```python
from build123d import *

# Parameters (mm, degrees)
SZKIC1_W                    = 90
SZKIC1_H                    = 56
DODANIE_WYCI_GNI_CIE1_DEPTH = 3
SZKIC2_W                    = 90
SZKIC2_H                    = 3
DODANIE_WYCI_GNI_CIE2_DEPTH = 34
SZKIC4_R                    = 1.75
WYTNIJ_WYCI_GNI_CIE1_DEPTH  = 81.808415403
ZAOKR_GLENIE1_R             = 5
SZKIC5_W                    = 46
SZKIC5_H                    = 40
WYTNIJ_WYCI_GNI_CIE2_DEPTH  = 81.808415403
SZKIC6_W                    = 3
SZKIC6_H                    = 50
DODANIE_WYCI_GNI_CIE4_DEPTH = 12
SZKIC7_W                    = 3
SZKIC7_H                    = 10
DODANIE_WYCI_GNI_CIE5_DEPTH = 10


with BuildPart() as part:
    # Szkic1 → Dodanie-wyciągnięcie1 (new body)
    with BuildSketch(Plane.XY):
        Rectangle(SZKIC1_W, SZKIC1_H)
    extrude(amount=DODANIE_WYCI_GNI_CIE1_DEPTH)

    # Szkic2 → Dodanie-wyciągnięcie2 (add)
    with BuildSketch(Plane.XY.offset(3)):
        with Locations((0, 26.5)):
            Rectangle(SZKIC2_W, SZKIC2_H)
        with Locations((0, -26.5)):
            Rectangle(SZKIC2_W, SZKIC2_H)
    extrude(amount=DODANIE_WYCI_GNI_CIE2_DEPTH)

    # Szkic4 → Wytnij-wyciągnięcie1 (cut, through all)
    with BuildSketch(Plane(origin=(0, 28, 0), x_dir=(1, 0, 0), z_dir=(0, 1, 0))):
        with Locations(Location((-40, -32, 0), (0, 0, 270))):
            Circle(SZKIC4_R)
        with Locations(Location((40, -32, 0), (0, 0, 270))):
            Circle(SZKIC4_R)
    extrude(amount=-WYTNIJ_WYCI_GNI_CIE1_DEPTH, mode=Mode.SUBTRACT)

    # Zaokrąglenie1
    zaokr_glenie1_edges = [part.edges().sort_by_distance(p)[0] for p in [
        (-45, 26.5, 37),
        (45, 26.5, 37),
        (45, -26.5, 37),
        (-45, -26.5, 37),
    ]]
    fillet(zaokr_glenie1_edges, radius=ZAOKR_GLENIE1_R)

    # Szkic5 → Wytnij-wyciągnięcie2 (cut, through all)
    with BuildSketch(Plane(origin=(0, 28, 0), x_dir=(1, 0, 0), z_dir=(0, 1, 0))):
        with Locations((0, -23)):
            Rectangle(SZKIC5_W, SZKIC5_H)
    extrude(amount=-WYTNIJ_WYCI_GNI_CIE2_DEPTH, mode=Mode.SUBTRACT)

    # Szkic6 → Dodanie-wyciągnięcie4 (add)
    with BuildSketch(Plane.XY.offset(3)):
        with Locations((-43.5, 0)):
            Rectangle(SZKIC6_W, SZKIC6_H)
        with Locations((43.5, 0)):
            Rectangle(SZKIC6_W, SZKIC6_H)
    extrude(amount=DODANIE_WYCI_GNI_CIE4_DEPTH)

    # Szkic7 → Dodanie-wyciągnięcie5 (add)
    with BuildSketch(Plane.XY.offset(15)):
        with Locations((-43.5, 20)):
            Rectangle(SZKIC7_W, SZKIC7_H)
        with Locations((-43.5, -20)):
            Rectangle(SZKIC7_W, SZKIC7_H)
        with Locations((43.5, -20)):
            Rectangle(SZKIC7_W, SZKIC7_H)
        with Locations((43.5, 20)):
            Rectangle(SZKIC7_W, SZKIC7_H)
    extrude(amount=DODANIE_WYCI_GNI_CIE5_DEPTH)


solid = part.part
```
Model file for the job. Use its own axes, mm. A direction names the side the tool comes from. Coordinates: 2 decimals unless noted, no trailing zeros. Write each loop counter-clockwise with the first axis right and the second up, starting at its lowest first coordinate (ties: lowest second). Pieces come first, ordered by that corner, then holes. Notation, with made-up numbers: (49, 40.5) - (99, 40.5) arc R20 ccw to (99, 46.5) - close; hole circle Ø3 at (78.25, -13). An arc over 180 degrees is marked (long way). Use a Markdown table: item, result. Add a question column.
Item 1: Band-saw the part on A-A, the plane z = 19. Write the cut outline in (x, y).
Item 2: 3-axis set-ups, long thin cutter, end or side, ignore diameter. For faces 1 (the face through (43, 20, 25)), 2 (the face through (-42, 0, 11)), 3 (the face through (-23, 27, 20)): which of +Z, -Z, +X, -X, +Y, -Y reach the whole face in a straight line?
Item 3: Drill centre lines: line 1 along X through (y, z) = (-26, 32); line 2 along Y through (x, z) = (36, 31.5); line 3 along X through (y, z) = (-17, 5). Where is each one in solid material? Low to high.
Item 4: Band-saw the part on C-C, the plane y = -17.5. Write the cut outline in (x, z).
Item 5: Two-plate mould, pull along Y, no slides. Class faces 4 (the face through (43, 15, 20)), 5 (the face through (-1, 28, 2)), 6 (the face through (23, 27, 20)): pulls with the +Y half, pulls with the -Y half, needs draft (parallel to the pull), parting line crosses it, or undercut.
Item 6: Drop a flat-ended pin along its axis: pin 1 (3.5 mm diameter, centred on x = -43, y = -22.5, fed in from +Z). Give the stop position or say it passes through.
Item 7: Band-saw the part on D-D, the plane x = -34. Write the cut outline in (y, z).
Item 8: Band-saw the part on B-B, the plane z = 12. Write the cut outline in (x, y).
A:
| question | item | result |
|---|---|---|
| 1 | outline | (-45, -28) - (-23, -28) - (-23, -25) - (-42, -25) - (-42, -15) - (-45, -15) - close; (-45, 15) - (-42, 15) - (-42, 25) - (-23, 25) - (-23, 28) - (-45, 28) - close; (23, -28) - (45, -28) - (45, -15) - (42, -15) - (42, -25) - (23, -25) - close; (23, 25) - (42, 25) - (42, 15) - (45, 15) - (45, 28) - (23, 28) - close |
| 2 | face 1 | +Z, +X, -X |
| 2 | face 2 | +Z |
| 2 | face 3 | +Z, +Y, -Y |
| 3 | line 1 | x = -45 to -41.75, -38.25 to -23, 23 to 38.25, 41.75 to 45 |
| 3 | line 2 | y = -28 to -25, 25 to 28 |
| 3 | line 3 | x = -45 to -42, 42 to 45 |
| 4 | outline | (-45, 0) - (45, 0) - (45, 25) - (42, 25) - (42, 3) - (-42, 3) - (-42, 25) - (-45, 25) - close |
| 5 | face 4 | undercut |
| 5 | face 5 | pulls with the +Y half |
| 5 | face 6 | needs draft |
| 6 | pin 1 | stops at z = 25 |
| 7 | outline | (-28, 0) - (28, 0) - (28, 37) - (25, 37) - (25, 3) - (-25, 3) - (-25, 37) - (-28, 37) - close |
| 8 | outline | (-45, -28) - (-23, -28) - (-23, -25) - (-42, -25) - (-42, 25) - (-23, 25) - (-23, 28) - (-45, 28) - close; (23, -28) - (45, -28) - (45, 28) - (23, 28) - (23, 25) - (42, 25) - (42, -25) - (23, -25) - close |
